```python
from build123d import *

# Parameters (mm, degrees)
SKETCH_1_W          = 32
SKETCH_1_H          = 338
EXTRUDE_1_DEPTH     = 5.5
SKETCH_2_W          = 10
SKETCH_2_H          = 5.5
CUT_EXTRUDE_1_DEPTH = 5.5
SKETCH_3_R          = 1.05
CUT_EXTRUDE_2_DEPTH = 10


with BuildPart() as part:
    # ｽｹｯﾁ1 → ﾎﾞｽ - 押し出し1 (new body)
    with BuildSketch(Plane.XY):
        with Locations((16, 169)):
            Rectangle(SKETCH_1_W, SKETCH_1_H)
    extrude(amount=EXTRUDE_1_DEPTH)

    # ｽｹｯﾁ2 → ｶｯﾄ - 押し出し1 (cut)
    with BuildSketch(Plane.XY.offset(5.5)):
        with Locations((16, 335.25)):
            Rectangle(SKETCH_2_W, SKETCH_2_H)
    extrude(amount=-CUT_EXTRUDE_1_DEPTH, mode=Mode.SUBTRACT)

    # ｽｹｯﾁ3 → ｶｯﾄ - 押し出し2 (cut)
    with BuildSketch(Plane.XY.offset(5.5)):
        with Locations((3, 5)):
            Circle(SKETCH_3_R)
        with Locations((29, 5)):
            Circle(SKETCH_3_R)
        with Locations((3, 33)):
            Circle(SKETCH_3_R)
        with Locations((29, 33)):
            Circle(SKETCH_3_R)
        with Locations((3, 61)):
            Circle(SKETCH_3_R)
        with Locations((29, 61)):
            Circle(SKETCH_3_R)
        with Locations((3, 89)):
            Circle(SKETCH_3_R)
        with Locations((29, 89)):
            Circle(SKETCH_3_R)
        with Locations((3, 117)):
            Circle(SKETCH_3_R)
        with Locations((29, 117)):
            Circle(SKETCH_3_R)
    extrude(amount=-CUT_EXTRUDE_2_DEPTH, mode=Mode.SUBTRACT)


solid = part.part
```
Check sheet for the modelled part. Datum: model origin and axes. Units: mm. A direction names the side the tool comes from. Coordinates: 2 decimals unless noted, no trailing zeros. Use a Markdown table: item, result.
1. Release check for a two-part mould opening along X. For faces 1 (the flat face through (16, 171, 0)), 2 (the flat face through (0, 167, 3)), 3 (the flat face through (21, 335, 3)) record: pulls with the +X half, pulls with the -X half, needs draft (parallel to the pull), parting line crosses it, or undercut.
Reported:
| item | result |
|---|---|
| face 1 | needs draft |
| face 2 | pulls with the -X half |
| face 3 | undercut |
2. Tool access check on faces 4 (the flat face through (16, 332.5, 3)), 5 (the flat face through (16, 171, 5.5)). Record the directions out of +Z, -Z, +X, -X, +Y, -Y that give a thin tool (end or side, any length) a straight path to the whole face; none if there is none.
Reported:
| item | result |
|---|---|
| face 4 | +Z, -Z, +Y |
| face 5 | +Z, +X, -X, +Y, -Y |
3. Go/stop test with flat-tipped pins: pin 1 Ø1.3 at (x, y) = (29, 33) entering from -Z; pin 2 Ø3 at (x, z) = (15.5, 2.5) entering from +Y. Record where each tip stops, or that it passes through.
Reported:
| item | result |
|---|---|
| pin 1 | passes through |
| pin 2 | stops at y = 332.5 |
4. Scan lines: line 1 along Y through (x, z) = (3, 3.45); line 2 along X through (y, z) = (117, 3.1); line 3 along Y through (x, z) = (3.5, 3.5). Record each from-to range of solid material in increasing order.
Reported:
| item | result |
|---|---|
| line 1 | y = 0 to 3.95, 6.05 to 31.95, 34.05 to 59.95, 62.05 to 87.95, 90.05 to 115.95, 118.05 to 338 |
| line 2 | x = 0 to 1.95, 4.05 to 27.95, 30.05 to 32 |
| line 3 | y = 0 to 4.08, 5.92 to 32.08, 33.92 to 60.08, 61.92 to 88.08, 89.92 to 116.08, 117.92 to 338 |
